```python
from build123d import *

# Parameters (mm, degrees)
BOSS_EXTRUDE1_DEPTH = 10
BOSS_EXTRUDE2_DEPTH = 32
BOSS_EXTRUDE3_DEPTH = 13
SKETCH4_R           = 2
CUT_EXTRUDE1_DEPTH  = 54.907327888
SKETCH5_R           = 2
CUT_EXTRUDE2_DEPTH  = 50.527769988
SKETCH6_R           = 4.5
CUT_EXTRUDE3_DEPTH  = 4
SKETCH7_R           = 4.5
CUT_EXTRUDE4_DEPTH  = 4
CHAMFER2_SIZE       = 2


with BuildPart() as part:
    # Sketch1 → Boss-Extrude1 (new body)
    with BuildSketch(Plane.XY):
        Polygon((0, 0), (0, -30), (-44, -30), (-44, -11), (-22, -11), (-22, 0), align=None)
    extrude(amount=BOSS_EXTRUDE1_DEPTH)

    # Sketch2 → Boss-Extrude2 (add)
    with BuildSketch(Plane.XY.offset(10)):
        Polygon((-44, -11), (-22, -11), (-22, -30), (-32, -30), (-32, -18), (-44, -18), align=None)
    extrude(amount=-BOSS_EXTRUDE2_DEPTH)

    # Sketch3 → Boss-Extrude3 (add)
    with BuildSketch(Plane.XY.offset(10)):
        Polygon((-44, -11), (-22, -11), (-22, 0), (-12, 0), (-12, -21), (-44, -21), align=None)
    extrude(amount=BOSS_EXTRUDE3_DEPTH)

    # Sketch4 → Cut-Extrude1 (cut, through all)
    with BuildSketch(Plane.XZ.offset(21)):
        with Locations(Location((-33, 16.5, 0), (0, 0, 270))):
            Circle(SKETCH4_R)
    extrude(amount=-CUT_EXTRUDE1_DEPTH, mode=Mode.SUBTRACT)

    # Sketch5 → Cut-Extrude2 (cut, through all)
    with BuildSketch(Plane.ZY.offset(32)):
        with Locations((-11, -24)):
            Circle(SKETCH5_R)
    extrude(amount=-CUT_EXTRUDE2_DEPTH, mode=Mode.SUBTRACT)

    # Sketch6 → Cut-Extrude3 (cut)
    with BuildSketch(Plane.ZY.offset(32)):
        with Locations((-11, -24)):
            Circle(SKETCH6_R)
    extrude(amount=-CUT_EXTRUDE3_DEPTH, mode=Mode.SUBTRACT)

    # Sketch7 → Cut-Extrude4 (cut)
    with BuildSketch(Plane.XZ.offset(21)):
        with Locations(Location((-33, 16.5, 0), (0, 0, 270))):
            Circle(SKETCH7_R)
    extrude(amount=-CUT_EXTRUDE4_DEPTH, mode=Mode.SUBTRACT)

    # Chamfer2
    chamfer2_edges = [part.edges().sort_by_distance(p)[0] for p in [
        (-28, -24, -13),
        (-33, -17, 18.5),
    ]]
    chamfer(chamfer2_edges, length=CHAMFER2_SIZE)

    # Mirror1: part across plane


with BuildPart() as part_1:
    add(part.part)
    add(part.part.mirror(Plane(origin=(0, 0, 10), x_dir=(0, 0, 1), z_dir=(0, -1, 0))))


solid = part_1.part
```
Work out the finished part from the listing and answer in its coordinate system (mm). A direction names the side the tool comes from. Round coordinates to 2 decimals unless told otherwise and drop trailing zeros. Loops run counter-clockwise (first coordinate to the right, second up) from the corner with the lowest first, then second, coordinate; pieces in that order, holes last. Notation, with made-up numbers: M 13,6 L 51,6 A28 cw 51,36 Z; hole C 10,-16 d8. An arc over 180 degrees is marked long. One line per question, with ' | ' between items.
Q1. Find section A-A, the plane x = -39. Give the vertices of the cut face in (y, z).
Conclusion:
outline: M -30,0 L -18,0 L -18,-22 L -11,-22 L -11,23 L -21,23 L -21,10 L -30,10 Z; M 11,-22 L 18,-22 L 18,0 L 30,0 L 30,10 L 21,10 L 21,23 L 11,23 Z
Q2. Find section D-D, the plane z = 16.5. Give the vertices of the cut face in (x, y), then the cut area to 3 significant figures.
Conclusion:
outline: M -44,-21 L -37.5,-21 L -37.5,-17 L -37,-17 L -35,-15 L -35,-11 L -44,-11 Z; M -44,11 L -35,11 L -35,15 L -37,17 L -37.5,17 L -37.5,21 L -44,21 Z; M -31,-15 L -29,-17 L -28.5,-17 L -28.5,-21 L -12,-21 L -12,21 L -28.5,21 L -28.5,17 L -29,17 L -31,15 L -31,11 L -22,11 L -22,-11 L -31,-11 Z | area: 732 mm2
Q3. The mould has two halves that part along X. Classify faces 4 (the flat face through (-28, 21, 16)), 5 (the cylindrical face through (-34.952, -13.028, 16.934)), 6 (the flat face through (-22, 20, -11)): +X half, -X half, draft (parallel to the pull), parting line (faces both ways), or undercut.
Conclusion:
face 4: draft | face 5: undercut | face 6: +X half
Q4. Find section C-C, the plane y = -24. Give the vertices of the cut face in (x, z).
Conclusion:
outline: M -44,0 L -32,0 L -32,-6.5 L -28,-6.5 L -28,-7 L -26,-9 L -22,-9 L -22,0 L 0,0 L 0,10 L -44,10 Z; M -32,-22 L -22,-22 L -22,-13 L -26,-13 L -28,-15 L -28,-15.5 L -32,-15.5 Z
Q5. Each of these flat-tipped pins is pushed along its axis until it touches: pin 1 Ø3.5 at (y, z) = (26, -6) entering from -X; pin 2 Ø4 at (x, z) = (-22.5, 13.5) entering from +Y; pin 3 Ø11 at (x, y) = (-8, 12.5) entering from -Z. Where does it stop, or does it pass through?
Conclusion:
pin 1: stops at x = -32 | pin 2: stops at y = 21 | pin 3: stops at z = 0
Q6. Consider line 1 along Y through (x, z) = (-24, -11); line 2 along Y through (x, z) = (-30.3, -11); line 3 along Z through (x, y) = (-24, 24). Determine where each line is inside the solid, lowest interval first. Write a range as from..to.
Conclusion:
line 1: y = -30..-26, -22..-11, 11..22, 26..30 | line 2: y = -30..-28.5, -19.5..-11, 11..19.5, 28.5..30 | line 3: z = -22..-13, -9..10
Q7. A tool of negligible diameter and unlimited length cuts with its end or side. For faces 1 (the flat face through (-28, 27, -14)), 2 (the flat face through (-32, 20, -8)), 3 (the flat face through (-38, -18, -11)), from which of +Z, -Z, +X, -X, +Y, -Y can it reach the whole face along a straight path? Write none if from no direction.
Conclusion:
face 1: -X | face 2: -Z, -X, +Y | face 3: -Z, -X, -Y
Q8. Find section B-B, the plane z = -1. Give the vertices of the cut face in (x, y), then the cut area to 3 significant figures.
Conclusion:
outline: M -44,-18 L -32,-18 L -32,-30 L -22,-30 L -22,-11 L -44,-11 Z; M -44,11 L -22,11 L -22,30 L -32,30 L -32,18 L -44,18 Z | area: 548 mm2
